Autodesk Fusion 360 part; units mm, degrees
sketch "Sketch1" plane through (0, 0, 0) normal (0, 0, 1) x (1, 0, 0)
  line L0 (0, 0) -> (8.5, 0)
  line L1 (8.5, 0) -> (8.5, 8.5)
  line L2 (8.5, 8.5) -> (0, 8.5)
  line L3 (0, 8.5) -> (0, 0)
  dimension "d1" = 8.5
extrude "Extrude1" add sketch "Sketch1" along normal blind 3
sketch "Sketch2" plane through (0, 0, 0) normal (0, 0, -1) x (1, 0, 0)
  line L0 (0, 0) -> (0, -8.5)
  line L1 (0, -8.5) -> (8.5, -8.5)
  line L2 (8.5, -8.5) -> (8.5, 0)
  line L3 (8.5, 0) -> (0, 0)
  line L4 (0.5, -0.5) -> (8, -0.5)
  line L5 (8, -0.5) -> (8, -8)
  line L6 (8, -8) -> (0.5, -8)
  line L7 (0.5, -8) -> (0.5, -0.5)
  line L8 (0.5, -0.5) -> (8, -8) construction
  line L9 (8.5, 0) -> (0, -8.5) construction
  dimension "d4" = 7.5
extrude "Extrude2" add sketch "Sketch2" along normal blind 17 contours L4 L5 L6 L7
sketch "Sketch3" plane through (8, 0, 0) normal (1, 0, 0) x (0, 1, 0)
  line L0 (8, 0) -> (0.5, 0)
  line L1 (0.5, 0) -> (0.5, -17)
  line L2 (0.5, -17) -> (8, -17)
  line L3 (8, -17) -> (8, 0)
  line L4 (0.5, -17) -> (4.25, -14.8349)
  line L5 (4.25, -14.8349) -> (8, -17)
  line L6 (8, -17) -> (0.5, -17)
  dimension "d7" = 120
extrude "Extrude3" cut sketch "Sketch3" against normal through all contours L2 L4 L5 L6
fillet "Fillet1" radius 1 2 edges at (4.25, 0.5, -17) (4.25, 8, -17)
Can you work these out from the model? Positions are in its coordinate system, mm. A direction names the side the tool comes from. Coordinates: 2 decimals unless noted, no trailing zeros. Loops run counter-clockwise (first coordinate to the right, second up) from the corner with the lowest first, then second, coordinate; pieces in that order, holes last. Notation, with made-up numbers: (44, 69) - (54, 69) arc R27 cw to (54, 96) - close; hole circle Ø10 at (58, 76.5). An arc over 180 degrees is marked (long way). Answer as CSV lines item,"result". Start each with the question number.
1) Thinking about a two-plate mould opening in Y: for faces 1 (the flat face through (4.3, 5.4, -15.5)), 2 (the flat face through (4, 4, 3)), 3 (the cylindrical face through (4.2, 7.51, -16.13)), 4 (the flat face through (4, 8.5, 1)), which applies, pulls with the +Y half, pulls with the -Y half, needs draft (parallel to the pull), parting line crosses it, or undercut?
2) Which directions (+Z, -Z, +X, -X, +Y, -Y) give clear straight access to the entire face, cutting with the end or side of a thin tool? Please do faces 5 (the flat face through (0.5, 4, -8)), 6 (the flat face through (8, 4, -8)), 7 (the flat face through (4, 0.5, -8)), 8 (the flat face through (4, 8, -8)), 9 (the flat face through (4.3, 3.1, -15.5)).
3) Suppose I cut it at D-D (y = 7.75). Please give me the cut outline in (x, z), plus the area to 3 significant figures.
4) Suppose I cut it at A-A (y = 1). Please give me the cut outline in (x, z).
5) For pin 1 (2 mm diameter, centred on y = 4, z = -13.5, fed in from +X); pin 2 (2.5 mm diameter, centred on x = 5, y = 4.5, fed in from -Z); pin 3 (1.5 mm diameter, centred on x = 3, z = -10.5, fed in from +Y), each with a flat end and sliding along its axis, tell me the tip position at first contact or that it passes through.
6) I need wall thicknesses on line 1 (X direction, y = 1.5, z = -2.5); line 2 (Z direction, x = 1.5, y = 8.25). Which ranges of each line are inside material? Lowest first, please. Write a range as from..to.
7) Suppose I cut it at C-C (z = -3.25). Please give me the cut outline in (x, y).
8) Suppose I cut it at B-B (x = 3.25). Please give me the cut outline in (y, z).
Check result:
1,face 1,"undercut"
1,face 2,"needs draft"
1,face 3,"undercut"
1,face 4,"pulls with the +Y half"
2,face 5,"-Z, -X, +Y, -Y"
2,face 6,"-Z, +X, +Y, -Y"
2,face 7,"-Z, +X, -X, -Y"
2,face 8,"-Z, +X, -X, +Y"
2,face 9,"-Z, +X, -X"
3,outline,"(0, 0) - (0.5, 0) - (0.5, -15.93) - (8, -15.93) - (8, 0) - (8.5, 0) - (8.5, 3) - (0, 3) - close"
3,area,"145 mm²"
4,outline,"(0, 0) - (0.5, 0) - (0.5, -16.13) - (8, -16.13) - (8, 0) - (8.5, 0) - (8.5, 3) - (0, 3) - close"
5,pin 1,"stops at x = 8"
5,pin 2,"stops at z = -15.7"
5,pin 3,"stops at y = 8"
6,line 1,"x = 0.5..8"
6,line 2,"z = 0..3"
7,outline,"(0.5, 0.5) - (8, 0.5) - (8, 8) - (0.5, 8) - close"
8,outline,"(0, 0) - (0.5, 0) - (0.5, -15.27) arc R1 ccw to (2, -16.13) - (4.25, -14.83) - (6.5, -16.13) arc R1 ccw to (8, -15.27) - (8, 0) - (8.5, 0) - (8.5, 3) - (0, 3) - close"
